Job drawing, mm, ordinate dimensions from the low corner. One solid piece. Give positions to 0.01 mm unless a question says otherwise; leave off trailing zeros. Order: outer loops, then holes, each group sorted by start corner. A loop starts at its lowest first (then second) coordinate and runs counter-clockwise, first axis right, second up. Notation, with made-up numbers: (-3.5, -9) - (51.5, -9) arc R18 cw to (51.5, 16) - close; hole circle Ø10 at (68.25, 69.25). An arc over 180 degrees is marked (long way). Write each question's results on one line, items separated by ' | '. Start each with the question number.
1) Drill centre lines: line 1 along Z through (x, y) = (3, 0.3) (1 decimal); line 2 along X through (y, z) = (0.6, 2.75) (1 decimal); line 3 along X through (y, z) = (2.2, 18). Where is each one in solid material? Low to high. Write a range as from..to.
2) Cut at D-D on x = 13. List the corners of the cut face in (y, z).
3) Cut at C-C on y = 1.25. List the corners of the cut face in (x, z) (1 decimal), plus the area to 3 significant figures.
4) Cut at A-A on x = 23.75. List the corners of the cut face in (y, z).
5) Drop a flat-ended pin along its axis: pin 1 Ø0.6 at (x, y) = (11.5, 2) entering from -Z. Give the stop position or say it passes through.
6) Cut at B-B on z = 12. List the corners of the cut face in (x, y).
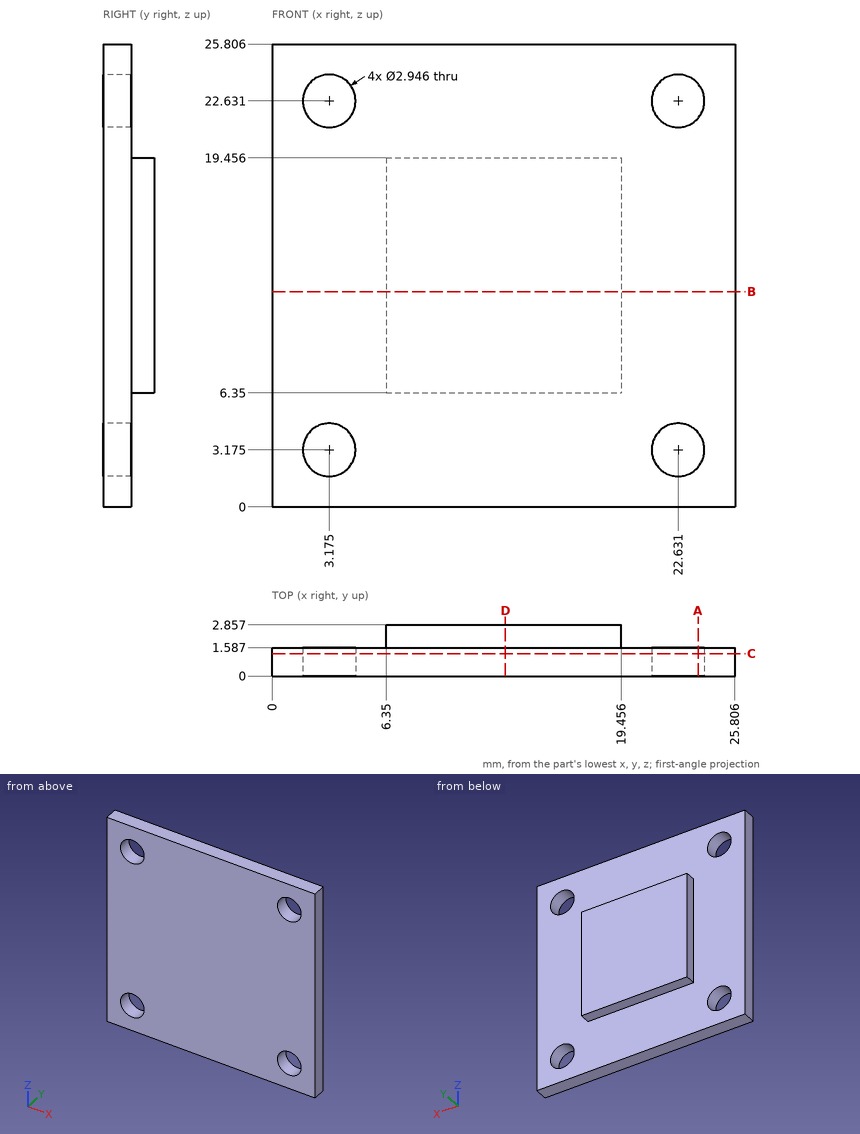
Results:
1) line 1: 0..1.7, 4.6..21.2, 24.1..25.8 | line 2: 0..1.8, 4.6..21.2, 24..25.8 | line 3: 6.35..19.46
2) outline: (0, 0) - (1.59, 0) - (1.59, 6.35) - (2.86, 6.35) - (2.86, 19.46) - (1.59, 19.46) - (1.59, 25.81) - (0, 25.81) - close
3) outline: (0, 0) - (25.8, 0) - (25.8, 25.8) - (0, 25.8) - close; hole circle Ø2.9 at (3.2, 3.2); hole circle Ø2.9 at (3.2, 22.6); hole circle Ø2.9 at (22.6, 3.2); hole circle Ø2.9 at (22.6, 22.6) | area: 639 mm^2
4) outline: (0, 0) - (1.59, 0) - (1.59, 2.22) - (0, 2.22) - close; (0, 4.13) - (1.59, 4.13) - (1.59, 21.67) - (0, 21.67) - close; (0, 23.59) - (1.59, 23.59) - (1.59, 25.81) - (0, 25.81) - close
5) pin 1: z = 6.35
6) outline: (0, 0) - (25.81, 0) - (25.81, 1.59) - (19.46, 1.59) - (19.46, 2.86) - (6.35, 2.86) - (6.35, 1.59) - (0, 1.59) - close
